Read the model definition and answer for the solid it produces. Units are mm, in the model's axes. A direction names the side the tool comes from. Give positions to 0.01 mm unless a question says otherwise; leave off trailing zeros. Write each loop counter-clockwise with the first axis right and the second up, starting at its lowest first coordinate (ties: lowest second). Pieces come first, ordered by that corner, then holes.
```python
from build123d import *

# Parameters (mm, degrees)
BOSS_EXTRUDE1_DEPTH = 100
BOSS_EXTRUDE2_DEPTH = 3
SKETCH4_W           = 71
SKETCH4_H           = 3
BOSS_EXTRUDE3_DEPTH = 20
BOSS_EXTRUDE4_REACH = 48
SKETCH6_W           = 48
SKETCH6_H           = 3
CUT_EXTRUDE1_DEPTH  = 3
SKETCH8_R           = 2.5
SKETCH8_R_2         = 1.7
CUT_EXTRUDE2_DEPTH  = 3
SKETCH9_R           = 3.2
SKETCH9_R_2         = 2.5
CUT_EXTRUDE3_DEPTH  = 3
SKETCH10_R          = 1.7
CUT_EXTRUDE4_DEPTH  = 3
SKETCH13_R          = 2.5
CUT_EXTRUDE6_DEPTH  = 3
BOSS_EXTRUDE5_DEPTH = 3
BOSS_EXTRUDE6_DEPTH = 5
CUT_EXTRUDE8_DEPTH  = 18
SKETCH20_W          = 20.000898322
SKETCH20_H          = 3
CUT_EXTRUDE9_DEPTH  = 3
SKETCH21_W          = 20.000898322
SKETCH21_H          = 3
CUT_EXTRUDE10_DEPTH = 3
SKETCH22_R          = 4.125
BOSS_EXTRUDE7_DEPTH = 3
LPATTERN1_COUNT     = 2
LPATTERN1_PITCH     = 28
LPATTERN2_COUNT     = 2
LPATTERN2_PITCH     = 164
LPATTERN3_COUNT     = 2
LPATTERN3_PITCH     = 136
SKETCH23_W          = 16
SKETCH23_H          = 53
CUT_EXTRUDE11_DEPTH = 3


with BuildPart() as part:
    # Sketch1 → Boss-Extrude1 (new body)
    with BuildSketch(Plane.XY):
        Polygon((0, 60), (0, -3), (3, -3), (3, 63), (-90, 63), (-90, 20), (-110.000898322, 20), (-110.033128512, 58.939230707), (-164, 48), (-164, -3), (-161, -3), (-161, 45.547095944), (-113, 55.276825673), (-113, 17), (-90, 17), (-90, -3), (-87, -3), (-87, 60), align=None)
    extrude(amount=BOSS_EXTRUDE1_DEPTH)

    # Sketch2 → Boss-Extrude2 (add)
    with BuildSketch(Plane.XY.offset(100)):
        Polygon((-164, -3), (3, -3), (3, 63), (-90, 63), (-90, 35.999994519), (-110.014141595, 35.999994519), (-110.033128512, 58.939230707), (-164, 48), align=None)
    extrude(amount=BOSS_EXTRUDE2_DEPTH)

    # Sketch4 → Boss-Extrude3 (add)
    with BuildSketch(Plane.XZ.offset(3)):
        with Locations((-125.5, 67.5)):
            Rectangle(SKETCH4_W, SKETCH4_H)
    extrude(amount=-BOSS_EXTRUDE3_DEPTH)

    # Boss-Extrude4: up to this face of the body (flat: up to its plane)
    boss_extrude4_end = Plane(part.part.faces().sort_by_distance((-137, 50.411960808, 50))[0])
    # Sketch6 → Boss-Extrude4 (add, up to the picked face)
    with BuildSketch(Plane(origin=(0, 17, 0), x_dir=(1, 0, 0), z_dir=(0, 1, 0)), mode=Mode.PRIVATE) as boss_extrude4_sk1:
        with Locations((-137, -67.5)):
            Rectangle(SKETCH6_W, SKETCH6_H)
    boss_extrude4_tool1 = split(extrude(boss_extrude4_sk1.sketch, amount=BOSS_EXTRUDE4_REACH, mode=Mode.PRIVATE), bisect_by=boss_extrude4_end, keep=Keep.BOTH, mode=Mode.PRIVATE)
    add(boss_extrude4_tool1.solids().sort_by_distance((-137, 17, 67.5))[0])

    # Sketch7 → Cut-Extrude1 (cut)
    with BuildSketch(Plane.ZY.offset(164)):
        with BuildLine():
            Line((37, 44), (37, 57))
            Line((37, 57), (63, 57))
            Line((63, 57), (63, 44))
            ThreePointArc((63, 44), (50, 31), (37, 44))
        make_face()
    extrude(amount=-CUT_EXTRUDE1_DEPTH, mode=Mode.SUBTRACT)

    # Sketch8 → Cut-Extrude2 (cut)
    with BuildSketch(Plane(origin=(0, 0, 66), x_dir=(-1, 0, 0), z_dir=(0, 0, -1))):
        with Locations((136, 22)):
            Circle(SKETCH8_R)
        with Locations((151.5, 37.5)):
            Circle(SKETCH8_R_2)
        with Locations((120.5, 37.5)):
            Circle(SKETCH8_R_2)
        with Locations((151.5, 6.5)):
            Circle(SKETCH8_R_2)
        with Locations((120.5, 6.5)):
            Circle(SKETCH8_R_2)
    extrude(amount=-CUT_EXTRUDE2_DEPTH, mode=Mode.SUBTRACT)

    # Sketch9 → Cut-Extrude3 (cut)
    with BuildSketch(Plane(origin=(-87, 0, 0), x_dir=(0, 0, -1), z_dir=(1, 0, 0))):
        with Locations((-31, 29.5)):
            Circle(SKETCH9_R)
        with Locations((-7.43, 53.07)):
            Circle(SKETCH9_R_2)
        with Locations((-7.43, 5.93)):
            Circle(SKETCH9_R_2)
        with Locations((-54.57, 53.07)):
            Circle(SKETCH9_R_2)
        with Locations((-54.57, 5.93)):
            Circle(SKETCH9_R_2)
    extrude(amount=-CUT_EXTRUDE3_DEPTH, mode=Mode.SUBTRACT)

    # Sketch10 → Cut-Extrude4 (cut)
    with BuildSketch(Plane(origin=(0, 0, 66), x_dir=(-1, 0, 0), z_dir=(0, 0, -1))):
        with Locations((99.5, 6.5)):
            Circle(SKETCH10_R)
    extrude(amount=-CUT_EXTRUDE4_DEPTH, mode=Mode.SUBTRACT)

    # Sketch13 → Cut-Extrude6 (cut)
    with BuildSketch(Plane.ZY.offset(90)):
        with Locations((94.5, 6.43)):
            Circle(SKETCH13_R)
    extrude(amount=-CUT_EXTRUDE6_DEPTH, mode=Mode.SUBTRACT)

    # Sketch14 → Boss-Extrude5 (add)
    with BuildSketch(Plane(origin=(0, 0, 0), x_dir=(-1, 0, 0), z_dir=(0, 0, -1))):
        Polygon((-3, 63), (-3, -3), (164, -3), (164, 48), (110.033128512, 58.939230707), (110.014141595, 35.999994519), (90, 35.999994519), (90, 63), align=None)
    extrude(amount=BOSS_EXTRUDE5_DEPTH)

    # Sketch15 → Boss-Extrude6 (add)
    with BuildSketch(Plane.XZ.offset(3)):
        with BuildLine():
            ThreePointArc((-159, 93), (-155.464466094, 94.464466094), (-154, 98))
            Line((-154, 98), (-154, 100))
            Line((-154, 100), (-159, 100))
            ThreePointArc((-159, 100), (-157.585786438, 99.414213562), (-157, 98))
            ThreePointArc((-157, 98), (-159, 96), (-161, 98))
            Line((-161, 98), (-161, 93))
            Line((-161, 93), (-159, 93))
        make_face()
        with BuildLine():
            ThreePointArc((-161, 98), (-160.414213562, 99.414213562), (-159, 100))
            Line((-159, 100), (-161, 100))
            Line((-161, 100), (-161, 98))
        make_face()
        with BuildLine():
            Line((-7, 100), (-7, 98))
            ThreePointArc((-7, 98), (-5.535533906, 94.464466094), (-2, 93))
            Line((-2, 93), (0, 93))
            Line((0, 93), (0, 98))
            ThreePointArc((0, 98), (-3.414213563, 96.585786438), (-1.999999999, 100))
            Line((-1.999999999, 100), (-7, 100))
        make_face()
        with BuildLine():
            Line((0, 100), (-1.999999999, 100))
            ThreePointArc((-1.999999999, 100), (-0.585786437, 99.414213562), (0, 98))
            Line((0, 98), (0, 100))
        make_face()
        with BuildLine():
            Line((0, 2), (0, 7))
            Line((0, 7), (-2, 7))
            ThreePointArc((-2, 7), (-5.535533906, 5.535533906), (-7, 2))
            Line((-7, 2), (-7, 0))
            Line((-7, 0), (-2, 0))
            ThreePointArc((-2, 0), (-3.414213562, 3.414213562), (0, 2))
        make_face()
        with BuildLine():
            Line((0, 0), (0, 2))
            ThreePointArc((0, 2), (-0.585786438, 0.585786438), (-2, 0))
            Line((-2, 0), (0, 0))
        make_face()
        with BuildLine():
            ThreePointArc((-154, 2), (-155.464466094, 5.535533906), (-159, 7))
            Line((-159, 7), (-161, 7))
            Line((-161, 7), (-161, 2))
            ThreePointArc((-161, 2), (-159, 4), (-157, 2))
            ThreePointArc((-157, 2), (-157.585786438, 0.585786438), (-159, 0))
            Line((-159, 0), (-154, 0))
            Line((-154, 0), (-154, 2))
        make_face()
        with BuildLine():
            ThreePointArc((-159, 0), (-160.414213562, 0.585786438), (-161, 2))
            Line((-161, 2), (-161, 0))
            Line((-161, 0), (-159, 0))
        make_face()
    extrude(amount=-BOSS_EXTRUDE6_DEPTH)

    # Sketch19 → Cut-Extrude8 (cut)
    with BuildSketch(Plane(origin=(0, 63, 0), x_dir=(1, 0, 0), z_dir=(0, 1, 0))):
        with BuildLine():
            Line((-136, -37), (-164, -37))
            Line((-164, -37), (-164, -63))
            Line((-164, -63), (-136, -63))
            ThreePointArc((-136, -63), (-123, -50), (-136, -37))
        make_face()
    extrude(amount=-CUT_EXTRUDE8_DEPTH, mode=Mode.SUBTRACT)

    # Sketch20 → Cut-Extrude9 (cut)
    with BuildSketch(Plane(origin=(0, 0, 100), x_dir=(-1, 0, 0), z_dir=(0, 0, -1))):
        with Locations((100.000449161, 21.5)):
            Rectangle(SKETCH20_W, SKETCH20_H)
    extrude(amount=-CUT_EXTRUDE9_DEPTH, mode=Mode.SUBTRACT)

    # Sketch21 → Cut-Extrude10 (cut)
    with BuildSketch(Plane.XY):
        with Locations((-100.000449161, 21.5)):
            Rectangle(SKETCH21_W, SKETCH21_H)
    extrude(amount=-CUT_EXTRUDE10_DEPTH, mode=Mode.SUBTRACT)

    # Sketch22 → Boss-Extrude7 (add)
    with BuildSketch(Plane.ZY.offset(164)):
        with BuildLine():
            Line((103, 0.500009795), (103, 24.5))
            Line((103, 24.5), (129.095417441, 18.252679991))
            ThreePointArc((129.095417441, 18.252679991), (135.937956019, 8.445029172), (127.000002345, 0.500009795))
            Line((127.000002345, 0.500009795), (103, 0.500009795))
        make_face()
        with Locations((127.000002345, 9.500009795)):
            Circle(SKETCH22_R, mode=Mode.SUBTRACT)
        with BuildLine():
            Line((-3, 24.5), (-29.095417441, 18.252679991))
            ThreePointArc((-29.095417441, 18.252679991), (-35.937956019, 8.445029172), (-27.000002345, 0.500009795))
            Line((-27.000002345, 0.500009795), (-3, 0.500009795))
            Line((-3, 0.500009795), (-3, 24.5))
        make_face()
        with Locations((-27.000002345, 9.500009795)):
            Circle(SKETCH22_R, mode=Mode.SUBTRACT)
    boss_extrude7 = extrude(amount=-BOSS_EXTRUDE7_DEPTH)

    # LPattern1: Boss-Extrude7 ×2
    with Locations(*[(i * LPATTERN1_PITCH, 0, 0) for i in range(1, LPATTERN1_COUNT)]):
        add(boss_extrude7)

    # LPattern2: Boss-Extrude7 ×2
    with Locations(*[(i * LPATTERN2_PITCH, 0, 0) for i in range(1, LPATTERN2_COUNT)]):
        add(boss_extrude7)

    # LPattern3: Boss-Extrude7 ×2
    with Locations(*[(i * LPATTERN3_PITCH, 0, 0) for i in range(1, LPATTERN3_COUNT)]):
        add(boss_extrude7)

    # Sketch23 → Cut-Extrude11 (cut)
    with BuildSketch(Plane(origin=(3, 0, 0), x_dir=(0, 0, -1), z_dir=(1, 0, 0))):
        with Locations((-76, 26.5)):
            Rectangle(SKETCH23_W, SKETCH23_H)
    extrude(amount=-CUT_EXTRUDE11_DEPTH, mode=Mode.SUBTRACT)


solid = part.part
```
Item 1: Determine the mould class of faces 1 (the flat face through (-44, 63, 51)), 2 (the flat face through (-25, 10, -16)) for opening direction X: pulls with the +X half, pulls with the -X half, needs draft (parallel to the pull), parting line crosses it, or undercut.
Result set:
face 1: needs draft
face 2: undercut
Item 2: Section A-A (z = -19) is taken. Write down the section's boundary in (x, y), and give its area (3 significant figures).
Result set:
outline: (-164, 0.5) - (-161, 0.5) - (-161, 20.67) - (-164, 20.67) - close; (-136, 0.5) - (-133, 0.5) - (-133, 20.67) - (-136, 20.67) - close; (-28, 0.5) - (-25, 0.5) - (-25, 20.67) - (-28, 20.67) - close; (0, 0.5) - (3, 0.5) - (3, 20.67) - (0, 20.67) - close
area: 242 mm2
Item 3: Find the intervals of material crossed by line 1 along Z through (x, y) = (-107, 6.5); line 2 along X through (y, z) = (8, 108.5); line 3 along X through (y, z) = (44, 13.5), in increasing order.
Result set:
line 1: z = -3 to 0, 66 to 69, 100 to 103
line 2: x = -164 to -161, -136 to -133, -28 to -25, 0 to 3
line 3: x = -164 to -161, -113 to -110.02, -90 to -87, 0 to 3
Item 4: Section C-C (z = 50) is taken. Write down the section's boundary in (x, y).
Result set:
outline: (-164, -3) - (-161, -3) - (-161, 31) - (-164, 31) - close; (-123, 53.25) - (-113, 55.28) - (-113, 17) - (-90, 17) - (-90, -3) - (-87, -3) - (-87, 60) - (0, 60) - (0, -3) - (3, -3) - (3, 63) - (-90, 63) - (-90, 20) - (-110, 20) - (-110.03, 58.94) - (-123, 56.31) - close
Item 5: Section B-B (x = -73.5) is taken. Write down the section's boundary in (y, z), and give its area (3 significant figures).
Result set:
outline: (-3, -3) - (63, -3) - (63, 103) - (-3, 103) - (-3, 100) - (60, 100) - (60, 0) - (-3, 0) - close
area: 696 mm2
Item 6: Section D-D (z = 22) is taken. Write down the section's boundary in (x, y), and give its area (3 significant figures).
Result set:
outline: (-164, -3) - (-161, -3) - (-161, 45.55) - (-113, 55.28) - (-113, 17) - (-90, 17) - (-90, -3) - (-87, -3) - (-87, 60) - (0, 60) - (0, -3) - (3, -3) - (3, 63) - (-90, 63) - (-90, 20) - (-110, 20) - (-110.03, 58.94) - (-164, 48) - close
area: 1,140 mm2
Item 7: Which of the six approach directions +Z, -Z, +X, -X, +Y, -Y give full straight-line access (tool end or side, diameter ignored) to faces 3 (the flat face through (-133, 10, -16)), 4 (the flat face through (-134, 20, 100)), 5 (the flat face through (-151, 49, 63)), 6 (the cylindrical face through (-5, -1, 6))?
Result set:
face 3: -Z, +Y, -Y
face 4: none
face 5: -X, +Y
face 6: -Y
Item 8: Each of these flat-tipped pins is pushed along its axis until it touches: pin 1 Ø5 at (y, z) = (9.5, -27) entering from -X; pin 2 Ø3.5 at (x, y) = (1.5, 30.5) entering from -Z; pin 3 Ø0.9 at (x, z) = (-162.5, -13) entering from -Y; pin 4 Ø10 at (x, z) = (-104.5, 63.5) entering from +Y. Where does it stop, or does it pass through?
Result set:
pin 1: passes through
pin 2: stops at z = -3
pin 3: stops at y = 0.5
pin 4: stops at y = 20
